from build123d import *

# Parameters (mm, degrees)
BOSS_EXTRUDE1_DEPTH      = 6.35
BOSS_EXTRUDE1_DEPTH_BACK = 6.35
CHAMFER1_SIZE            = 6.35


with BuildPart() as part:
    # Sketch1 → Boss-Extrude1 (new, two sides: drawn at the far end of the back side and taken through both)
    with BuildSketch(Plane.XY.offset(-BOSS_EXTRUDE1_DEPTH_BACK)):
        with BuildLine():
            Line((536.695979739, 136.254867707), (560.943105898, 105.436216324))
            ThreePointArc((560.943105898, 105.436216324), (561.714171823, 104.617286319), (562.617631945, 103.947249887))
            Line((562.617631945, 103.947249887), (569.277605982, 99.869101199))
            ThreePointArc((569.277605982, 99.869101199), (570.871029516, 99.172603505), (572.593645863, 98.934484797))
            Line((572.593645863, 98.934484797), (615.194822187, 98.934484797))
            ThreePointArc((615.194822187, 98.934484797), (618.300590104, 98.123140378), (620.612705276, 95.896439332))
            Line((620.612705276, 95.896439332), (637.800986726, 67.778873585))
            ThreePointArc((637.800986726, 67.778873585), (638.081311904, 67.269225698), (638.313826657, 66.736065249))
            Line((638.313826657, 66.736065249), (648.207776972, 40.876876924))
            ThreePointArc((648.207776972, 40.876876924), (648.521355002, 39.761509046), (648.627053953, 38.607730725))
            Line((648.627053953, 38.607730725), (648.627053953, 28.543161139))
            ThreePointArc((648.627053953, 28.543161139), (648.864523478, 26.822849773), (649.559170865, 25.231206604))
            Line((649.559170865, 25.231206604), (652.382425554, 20.612766444))
            Line((652.382425554, 20.612766444), (656.038853698, 14.631373886))
            Line((656.038853698, 14.631373886), (675.181083361, 29.691866048))
            Line((675.181083361, 29.691866048), (625.044285009, 111.708484642))
            Line((625.044285009, 111.708484642), (577.280315143, 109.804848162))
            ThreePointArc((577.280315143, 109.804848162), (574.71471638, 110.235943554), (572.537308132, 111.659682846))
            Line((572.537308132, 111.659682846), (569.268870721, 114.928120257))
            ThreePointArc((569.268870721, 114.928120257), (568.444852538, 115.94228087), (567.845871294, 117.103637483))
            Line((567.845871294, 117.103637483), (560.349390782, 136.254867707))
            Line((560.349390782, 136.254867707), (536.695979739, 136.254867707))
        make_face()
    extrude(amount=BOSS_EXTRUDE1_DEPTH + BOSS_EXTRUDE1_DEPTH_BACK)

    # Chamfer1
    chamfer1_edges = [part.edges().sort_by_distance(p)[0] for p in [
        (574.71471638, 110.235943554, 6.35),
        (570.903089427, 113.293901552, 6.35),
        (601.162300076, 110.756666402, 6.35),
        (568.444852538, 115.94228087, 6.35),
        (564.097631038, 126.679252595, 6.35),
    ]]
    chamfer(chamfer1_edges, length=CHAMFER1_SIZE)


solid = part.part
Check sheet for the modelled part. Datum: model origin and axes. Units: mm. A direction names the side the tool comes from. Give positions to 0.01 mm unless a question says otherwise; leave off trailing zeros. Loops run counter-clockwise (first coordinate to the right, second up) from the corner with the lowest first, then second, coordinate; pieces in that order, holes last. Notation, with made-up numbers: M 65.5,-3.75 L 105.5,-3.75 A12 cw 105.5,0.25 Z; hole C 62.5,56 d11. An arc over 180 degrees is marked long. Answer as a JSON object with one key per item and string values. Group by question number.
Q1. Cross-section at C-C on y = 35.5. Record the cut outline in (x, z).
Q2. Material ranges on line 1 along X through (y, z) = (23.5, -1.5); line 2 along Y through (x, z) = (651, -4.5); line 3 along Y through (x, z) = (655, -1.5), recorded low to high. Write a range as [from, to].
Q3. Go/stop test with flat-tipped pins: P1, Ø3, axis at x = 590.5, z = 4.5, coming from the -Y side; P2, Ø1.5, axis at y = 65.5, z = -2, coming from the +X side; P3, Ø3, axis at y = 35.5, z = -2.5, coming from the -X side. Record where each tip stops, or that it passes through.
Q4. Access from +Z, -Z, +X, -X, +Y, -Y to the whole of each face (thin tool, end or side, straight path). Record for faces 1 (the flat face through (648.627, 34, 0)), 2 (the flat face through (650.46, 70.13, -0.09)).
Q5. Cross-section at B-B on x = 607.5. Record the cut outline in (y, z).
Q6. Cross-section at D-D on z = 4.25. Record the cut outline in (x, y), then the cut area to 3 significant figures.
Q7. Release check for a two-part mould opening along X. For faces 3 (the cylindrical face through (570.85, 99.18, -0.09)), 4 (the conical face through (565.766, 114.157, 3.219)), 5 (the flat face through (626, 89, -6.35)), 6 (the conical face through (573.59, 107.22, 3.22)) record: released by +X, released by -X, zero draft, split by the parting line, or undercut.
Q8. Cross-section at A-A on z = -4.75. Record the cut outline in (x, y).
Evaluation:
{
 "1": {"outline": "M 648.63,-6.35 L 671.63,-6.35 L 671.63,6.35 L 648.63,6.35 Z"},
 "2": {"line 1": "x = [650.62, 667.31]", "line 2": "y = [22.87, 69.25]", "line 3": "y = [16.33, 62.71]"},
 "3": {"P1": "stops at y = 98.93", "P2": "stops at x = 653.75", "P3": "stops at x = 648.63"},
 "4": {"face 1": "+Z, -Z, -X, -Y", "face 2": "+Z, -Z, +X, +Y"},
 "5": {"outline": "M 98.93,-6.35 L 111.01,-6.35 L 111.01,0 L 104.65,6.35 L 98.93,6.35 Z"},
 "6": {"outline": "M 536.7,136.25 L 560.94,105.44 A6.35 ccw 562.62,103.95 L 569.28,99.87 A6.35 ccw 572.59,98.93 L 615.19,98.93 A6.35 cw 620.61,95.9 L 637.8,67.78 A6.35 cw 638.31,66.74 L 648.21,40.88 A6.35 cw 648.63,38.61 L 648.63,28.54 A6.35 ccw 649.56,25.23 L 656.04,14.63 L 675.18,29.69 L 627.58,107.56 L 577.45,105.56 A10.6 cw 569.53,108.65 L 566.26,111.92 A10.6 cw 563.89,115.55 L 555.79,136.25 Z", "area": "2,280 mm2"},
 "7": {"face 3": "released by -X", "face 4": "released by +X", "face 5": "zero draft", "face 6": "undercut"},
 "8": {"outline": "M 536.7,136.25 L 560.94,105.44 A6.35 ccw 562.62,103.95 L 569.28,99.87 A6.35 ccw 572.59,98.93 L 615.19,98.93 A6.35 cw 620.61,95.9 L 637.8,67.78 A6.35 cw 638.31,66.74 L 648.21,40.88 A6.35 cw 648.63,38.61 L 648.63,28.54 A6.35 ccw 649.56,25.23 L 656.04,14.63 L 675.18,29.69 L 625.04,111.71 L 577.28,109.8 A6.35 cw 572.54,111.66 L 569.27,114.93 A6.35 cw 567.85,117.1 L 560.35,136.25 Z"}
}
